Could you check a few things on this drawing? It's one solid part, dimensions in mm from its lowest x, y, z. Round coordinates to 2 decimals unless told otherwise and drop trailing zeros. Write each loop counter-clockwise with the first axis right and the second up, starting at its lowest first coordinate (ties: lowest second). Pieces come first, ordered by that corner, then holes. Notation, with made-up numbers: (64.5, 28) -> (111.5, 28) arc R10 ccw to (111.5, 45) -> close; hole circle Ø4 at (68, 50). An arc over 180 degrees is marked (long way). Answer in a Markdown table with one row per item.
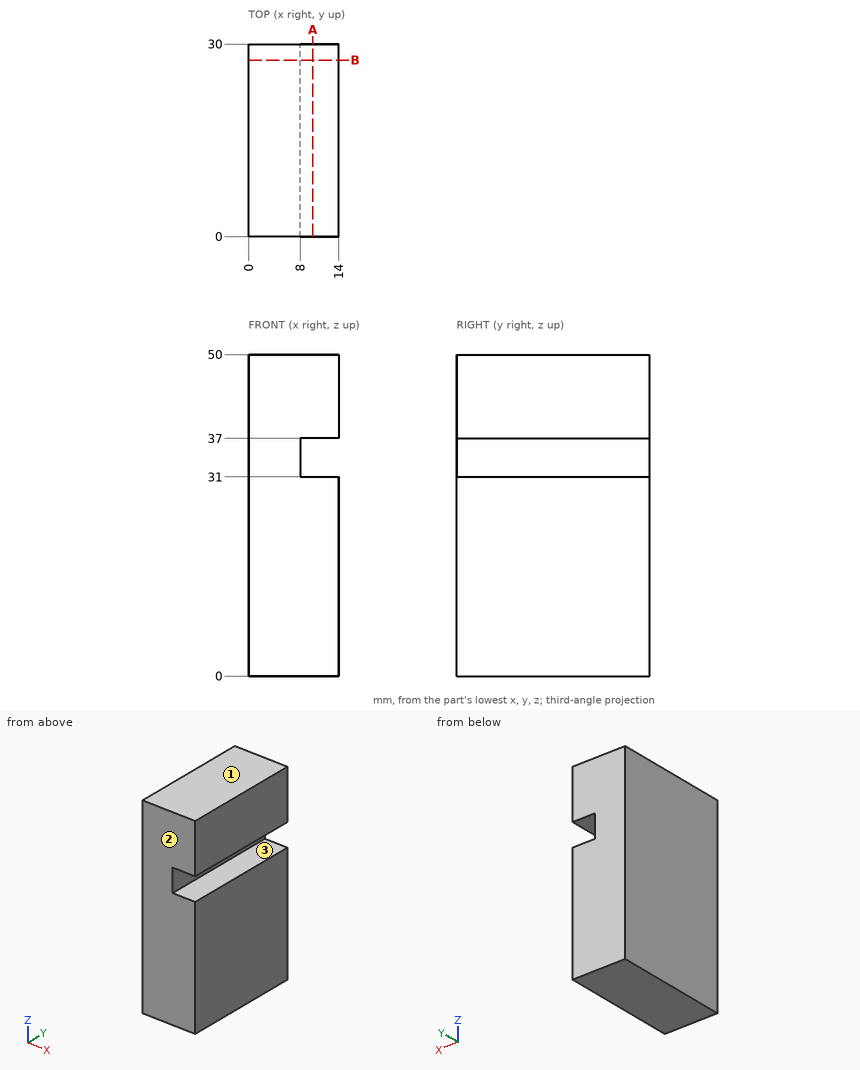
1) For pin 1 (5 mm diameter, centred on y = 21.5, z = 34, fed in from +X); pin 2 (1.5 mm diameter, centred on x = 9, z = 35, fed in from +Y), each with a flat end and sliding along its axis, tell me the tip position at first contact or that it passes through.
Findings:
| item | result |
|---|---|
| pin 1 | stops at x = 8 |
| pin 2 | passes through |
2) Please list where these lines run through material, in increasing order: line 1 (Z direction, x = 10.25, y = 13.5); line 2 (X direction, y = 18, z = 32.5).
Findings:
| item | result |
|---|---|
| line 1 | z = 0 to 31, 37 to 50 |
| line 2 | x = 0 to 8 |
3) Thinking about a two-plate mould opening in Z: for the marked faces 1, 2 and 3, which applies, +Z half, -Z half, draft (parallel to the pull), parting line (faces both ways), or undercut?
Findings:
| item | result |
|---|---|
| face 1 | +Z half |
| face 2 | draft |
| face 3 | undercut |
4) Imagine slicing it at A-A, the plane x = 10. Please give me the cut outline in (y, z), plus the area to 3 significant figures.
Findings:
| item | result |
|---|---|
| outline | (0, 0) -> (30, 0) -> (30, 31) -> (0, 31) -> close; (0, 37) -> (30, 37) -> (30, 50) -> (0, 50) -> close |
| area | 1,320 mm^2 |
5) Imagine slicing it at B-B, the plane y = 27.5. Please give me the cut outline in (x, z).
Findings:
| item | result |
|---|---|
| outline | (0, 0) -> (14, 0) -> (14, 31) -> (8, 31) -> (8, 37) -> (14, 37) -> (14, 50) -> (0, 50) -> close |
